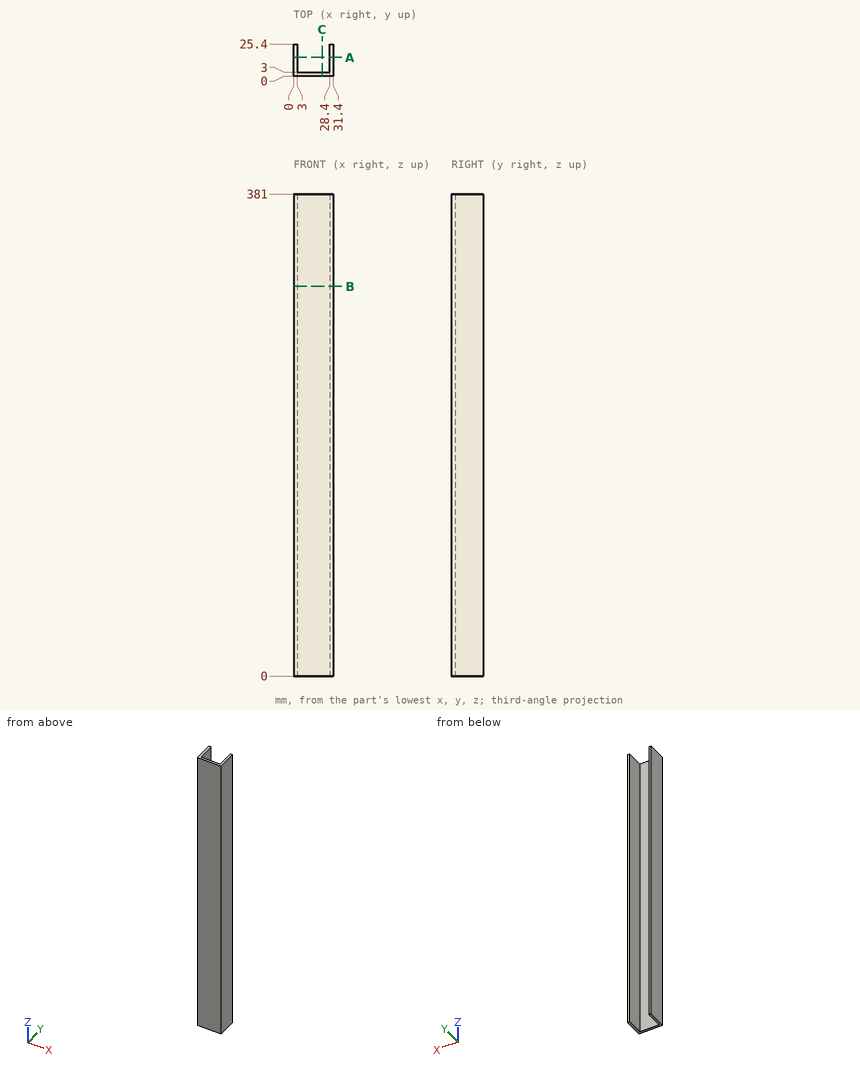
Check sheet for the drawn part. Datum: minimum x, y, z corner. Units: mm. Coordinates: 2 decimals unless noted, no trailing zeros. Write each loop counter-clockwise with the first axis right and the second up, starting at its lowest first coordinate (ties: lowest second). Pieces come first, ordered by that corner, then holes. Notation, with made-up numbers: (-7, -36) - (-3, -36) arc R23 cw to (-3, -21) - close; hole circle Ø4 at (-32, -23.5). An arc over 180 degrees is marked (long way). Answer as a JSON object with one key per item and string values.
(1) Thickness scan on line 1 along X through (y, z) = (5, 81.5); line 2 along Y through (x, z) = (28, 302.5). Record the ranges inside material, lowest first.
Report:
{"line 1": "0 to 3, 28.4 to 31.4", "line 2": "0 to 3"}
(2) Gauge pin test, flat end, axial feed: pin 1 Ø7.5 at (x, z) = (14, 255) entering from +Y. Record the tip position at first contact, or that the pin passes through.
Report:
{"pin 1": "y = 3"}
(3) Cross-section at C-C on x = 22.5. Record the cut outline in (y, z), plus the area to 3 significant figures.
Report:
{"outline": "(0, 0) - (3, 0) - (3, 381) - (0, 381) - close", "area": "1,140 mm^2"}
(4) Cross-section at A-A on y = 14.75. Record the cut outline in (x, z).
Report:
{"outline": "(0, 0) - (3, 0) - (3, 381) - (0, 381) - close; (28.4, 0) - (31.4, 0) - (31.4, 381) - (28.4, 381) - close"}
(5) Cross-section at B-B on z = 308. Record the cut outline in (x, y), plus the area to 3 significant figures.
Report:
{"outline": "(0, 0) - (31.4, 0) - (31.4, 25.4) - (28.4, 25.4) - (28.4, 3) - (3, 3) - (3, 25.4) - (0, 25.4) - close", "area": "229 mm^2"}
